Autodesk Inventor part; units mm, degrees
ref_plane "YZ Plane" through (0, 0, 0) normal (1, 0, 0) x (0, 1, 0)
ref_plane "XZ Plane" through (0, 0, 0) normal (0, 1, 0) x (-1, 0, 0)
ref_plane "XY Plane" through (0, 0, 0) normal (0, 0, 1) x (1, 0, 0)
sketch "Sketch1" plane through (0, 0, 0) normal (0, 1, 0) x (-1, 0, 0)
  line L0 (0, 0) -> (31.75, 0)
  line L1 (31.75, 0) -> (31.75, -82.55)
  line L2 (31.75, -82.55) -> (0, -82.55)
  line L3 (0, -82.55) -> (0, 0)
  line L4 (31.75, -82.55) -> (28.575, -82.55)
  line L5 (0, -82.55) -> (3.175, -82.55)
  line L6 (3.175, -82.55) -> (0, -82.55)
  line L7 (0, -82.55) -> (0, 0)
  line L8 (0, 0) -> (3.175, 0)
  line L9 (3.175, 0) -> (3.175, -82.55)
  line L10 (28.575, -82.55) -> (31.75, -82.55)
  line L11 (31.75, -82.55) -> (31.75, 0)
  line L12 (31.75, 0) -> (28.575, 0)
  line L13 (28.575, 0) -> (28.575, -82.55)
  line L14 (15.875, 0) -> (15.875, -6.35)
  circle A0 centre (15.875, -6.35) radius 2.1082
  line L15 (15.875, -6.35) -> (15.875, -71.3232)
  circle A1 centre (15.875, -71.3232) radius 5.715
  dimension "d0" = 31.75
  dimension "d1" = 3.175
  dimension "d2" = 3.175
  dimension "d3" = 82.55
  dimension "d4" = 6.35
  dimension "d5" = 4.2164
  dimension "d6" = 64.9732
  dimension "d13" = 11.43
extrude "Extrusion1" add sketch "Sketch1" along normal blind 6.35
sketch "Sketch2" plane through (0, 6.35, 0) normal (0, 1, 0) x (1, 0, 0)
  line L0 (-31.75, 0) -> (0, 0)
  line L1 (-31.75, 0) -> (-28.575, 0)
  line L2 (0, 0) -> (-3.175, 0)
  line L3 (0, 82.55) -> (-31.75, 82.55)
  line L4 (-28.575, 0) -> (-31.75, 0)
  line L5 (-31.75, 0) -> (-31.75, 82.55)
  line L6 (-31.75, 82.55) -> (-28.575, 82.55)
  line L7 (-28.575, 82.55) -> (-28.575, 0)
  line L8 (-3.175, 0) -> (0, 0)
  line L9 (0, 0) -> (0, 82.55)
  line L10 (0, 82.55) -> (-3.175, 82.55)
  line L11 (-3.175, 82.55) -> (-3.175, 0)
  dimension "d9" = 3.175
  dimension "d10" = 3.175
extrude "Extrusion2" add sketch "Sketch2" along normal blind 1.5875 contours L5 L3 L7 L0 | L11 L3 L9 L0
sketch "Sketch3" plane through (0, 0, 0) normal (0, -1, 0) x (1, 0, 0)
  line L0 (-31.75, -82.55) -> (-31.75, 0)
  line L1 (-31.75, -82.55) -> (-16.4111, -93.2904)
  line L2 (0, -82.55) -> (-31.75, -82.55)
  line L3 (-16.4111, -93.2904) -> (23.1212, -120.9712)
  line L4 (23.1212, -120.9712) -> (37.6901, -100.1648)
  line L5 (37.6901, -100.1648) -> (0, -73.7739)
  line L6 (0, 0) -> (0, -82.55)
  line L7 (-31.75, -82.55) -> (0, -82.55)
  dimension "d14" = 35
  dimension "d15" = 48.26
  dimension "d16" = 25.4
extrude "Extrusion3" add sketch "Sketch3" against normal blind 6.35
sketch "Sketch4" plane through (-31.75, 0, -82.55) normal (-0.5735764, 0, -0.819152) x (-0.819152, 0, 0.5735764)
  line L0 (-20.9743, 6.35) -> (-66.9854, 6.35)
  line L1 (0, 0) -> (0, 6.35)
  line L2 (-66.9854, 6.35) -> (0, 6.35)
  line L3 (0, 6.35) -> (0, 0)
  line L4 (0, 0) -> (-66.9854, 0)
  line L5 (-66.9854, 0) -> (-66.9854, 6.35)
  point P0 (21.3407, 0)
  point P1 (-20.9743, 6.35)
extrude "Extrusion4" add sketch "Sketch4" along normal blind 6.35
sketch "Sketch5" plane through (0, 0, 0) normal (0, -1, 0) x (1, 0, 0)
  circle A0 centre (-15.875, -71.3232) radius 5.715
  arc A1 (-31.75, -51.3533) -> (-35.3922, -87.7516) centre (-15.875, -71.3232) ccw
  line L0 (-31.75, -82.55) -> (-31.75, 0)
  line L1 (-31.75, -82.55) -> (-35.3922, -87.7516)
  line L2 (-31.75, -51.3533) -> (-31.75, -82.55)
  line L3 (-31.75, -82.55) -> (-35.3922, -87.7516)
  point P0 (0, 0)
extrude "Extrusion5" add sketch "Sketch5" against normal blind 6.35 contours L0 L1 A1
fillet "Fillet2" radius 3.175 3 edges at (0, 3.175, -73.7739) (19.479, 3.175, -126.1729) (37.6901, 3.175, -100.1648)
properties part number "intake sleds"
For this review, take the finished solid that the model builds, in its own axes (mm). Round coordinates to 2 decimals unless told otherwise and drop trailing zeros. Loops run counter-clockwise (first coordinate to the right, second up) from the corner with the lowest first, then second, coordinate; pieces in that order, holes last.
(1) We need section B-B (x = 29). Give the boundary of the cut face in (y, z), plus the area to 3 significant figures.
Returned:
outline: (0, -112.58) - (6.35, -112.58) - (6.35, -94.08) - (0, -94.08) - close
area: 117 mm2
(2) Mouldability with a two-part tool opening along Z and no side actions: class faces 1 (the cylindrical face through (-15.13, 3.13, -76.99)), 2 (the flat face through (-31.75, 4, -32)), 3 (the cylindrical face through (36.39, 3.22, -100.36)) as released by +Z, released by -Z, zero draft, split by the parting line, or undercut.
Returned:
face 1: undercut
face 2: zero draft
face 3: split by the parting line
(3) Wall thickness on line 1 along X through (y, z) = (3.5, -6.35); line 2 along X through (y, z) = (7, -78) (3 decimals); line 3 along Z through (x, y) = (-16.5, 2.75): over which ranges is each line inside the solid? List them lowest first.
Returned:
line 1: x = -31.75 to -17.98, -13.77 to 0
line 2: x = -31.75 to -28.575, -3.175 to 0
line 3: z = -100.98 to -77, -65.64 to -8.36, -4.34 to 0
(4) Clearance check with flat-ended pins moving along their axes: P1, Ø1, axis at x = 12.5, y = 5, coming from the +Z side; P2, Ø1.3, axis at y = 7.5, z = -54, coming from the +X side; P3, Ø4, axis at y = 4, z = -48.5, coming from the -X side. State where each tip first meets the part, or that it passes through.
Returned:
P1: stops at z = -82.18
P2: stops at x = 0
P3: stops at x = -31.75
(5) We need section D-D (x = -26.5). Give the boundary of the cut face in (y, z).
Returned:
outline: (0, -93.98) - (6.35, -93.98) - (6.35, 0) - (0, 0) - close
